from build123d import *

# Parameters (mm, degrees)
SKETCH_1_W               = 5
SKETCH_1_H               = 115
EXTRUDE_1_DEPTH          = 30
EXTRUDE_1_2_DEPTH        = 30
SKETCH_1_3_W             = 37.4
SKETCH_1_3_H             = 115
SKETCH_1_3_W_2           = 30.2
SKETCH_1_3_W_3           = 5
EXTRUDE_2_DEPTH          = 5
CUT_EXTRUDE_1_DEPTH      = 22.5
RIB_1_REACH              = 88.675
SKETCH_4_WALL_W          = 214.94733798
SKETCH_4_WALL_H          = 5
RIB_2_REACH              = 119.1
SKETCH_7_WALL_W          = 265.932906068
SKETCH_7_WALL_H          = 5
MIRROR_3_COPY_1_REACH    = 119.1
MIRROR_3_COPY_1_SKETCH_W = 265.932906068
MIRROR_3_COPY_1_SKETCH_H = 5


with BuildPart() as part:
    # Sketch 1 → Extrude 1 (new body)
    with BuildSketch(Plane.XY):
        with Locations((-17.6, 0)):
            Rectangle(SKETCH_1_W, SKETCH_1_H)
    extrude(amount=-EXTRUDE_1_DEPTH)



with BuildPart() as body_2:
    # Sketch 1 → Extrude 1 2 (new body)
    with BuildSketch(Plane.XY):
        with Locations((17.6, 0)):
            Rectangle(SKETCH_1_W, SKETCH_1_H)
    extrude(amount=-EXTRUDE_1_2_DEPTH)


with BuildPart() as part_1:
    add(part.part)

    add(body_2.part)  # Extrude 2 merges body 2
    # Sketch 1_3 → Extrude 2 (add)
    with BuildSketch(Plane.XY):
        with Locations((-38.8, 0)):
            Rectangle(SKETCH_1_3_W, SKETCH_1_3_H)
        Rectangle(SKETCH_1_3_W_2, SKETCH_1_3_H)
        with Locations((-17.6, 0)):
            Rectangle(SKETCH_1_3_W_3, SKETCH_1_3_H)
        with Locations((17.6, 0)):
            Rectangle(SKETCH_1_3_W_3, SKETCH_1_3_H)
        with Locations((38.8, 0)):
            Rectangle(SKETCH_1_3_W, SKETCH_1_3_H)
    extrude(amount=EXTRUDE_2_DEPTH)

    # Sketch 3 → Cut-Extrude 1 (cut, symmetric)
    with BuildSketch(Plane(origin=(0, 0, 0), x_dir=(0, 0, -1), z_dir=(1, 0, 0))):
        with BuildLine():
            Line((15, 24), (30, 24))
            Line((30, 24), (30, 16))
            Line((30, 16), (15, 16))
            ThreePointArc((15, 16), (11, 20), (15, 24))
        make_face()
        with BuildLine():
            Line((30, -16), (30, -24))
            Line((30, -24), (15, -24))
            ThreePointArc((15, -24), (11, -20), (15, -16))
            Line((15, -16), (30, -16))
        make_face()
    extrude(amount=CUT_EXTRUDE_1_DEPTH, both=True, mode=Mode.SUBTRACT)

    # Sketch 4 wall → Rib 1 (add, up to next)
    with BuildSketch(Plane(origin=(34, 0, -14), x_dir=(0.707106781187, 0, 0.707106781187), z_dir=(0.707106781187, 0, -0.707106781187)), mode=Mode.PRIVATE) as rib_1_sk1:
        Rectangle(SKETCH_4_WALL_W, SKETCH_4_WALL_H)
    rib_1_tool1 = extrude(rib_1_sk1.sketch, amount=-RIB_1_REACH, mode=Mode.PRIVATE) - part_1.part
    rib_1 = rib_1_tool1.solids().sort_by_distance((34, 0, -14))[0]
    add(rib_1)

    # Sketch 7 wall → Rib 2 (add, up to next)
    with BuildSketch(Plane(origin=(25, 40, -14), x_dir=(0.336336396998, 0, 0.941741911595), z_dir=(0.941741911595, 0, -0.336336396998)), mode=Mode.PRIVATE) as rib_2_sk1:
        Rectangle(SKETCH_7_WALL_W, SKETCH_7_WALL_H)
    rib_2_tool1 = extrude(rib_2_sk1.sketch, amount=-RIB_2_REACH, mode=Mode.PRIVATE) - part_1.part
    rib_2 = rib_2_tool1.solids().sort_by_distance((25, 40, -14))[0]
    add(rib_2)

    # Mirror 1: Rib 1 across plane
    add(rib_1.mirror(Plane.ZY))

    # Mirror 2: Rib 2 across plane
    add(rib_2.mirror(Plane.ZY))

    # Mirror 3: Rib 2 across plane
    add(rib_2.mirror(Plane(origin=(0, 0, 0), x_dir=(0, 0, 1), z_dir=(0, -1, 0))))

    # Mirror 3 copy 1 sketch → Mirror 3 copy 1 (add, up to next)
    with BuildSketch(Plane(origin=(-25, -40, -14), x_dir=(-0.336336396998, 0, 0.941741911595), z_dir=(-0.941741911595, 0, -0.336336396998)), mode=Mode.PRIVATE) as mirror_3_copy_1_sk1:
        Rectangle(MIRROR_3_COPY_1_SKETCH_W, MIRROR_3_COPY_1_SKETCH_H)
    mirror_3_copy_1_tool1 = extrude(mirror_3_copy_1_sk1.sketch, amount=-MIRROR_3_COPY_1_REACH, mode=Mode.PRIVATE) - part_1.part
    add(mirror_3_copy_1_tool1.solids().sort_by_distance((-25, -40, -14))[0])


solid = part_1.part
Model file for the job. Use its own axes, mm. A direction names the side the tool comes from. Coordinates: 2 decimals unless noted, no trailing zeros. Write each loop counter-clockwise with the first axis right and the second up, starting at its lowest first coordinate (ties: lowest second). Pieces come first, ordered by that corner, then holes. Notation, with made-up numbers: (24, 53.5) - (66, 53.5) arc R16 ccw to (66, 74.5) - close; hole circle Ø3 at (-29, 85). An arc over 180 degrees is marked (long way). Write each question's results on one line, items separated by ' | '. Start each with the question number.
1) Cut at B-B (y = 12). Write the cut outline in (x, z), then the cut area to 3 significant figures.
2) 3-axis set-ups, long thin cutter, end or side, ignore diameter. For faces 1 (the face through (24, 37.5, -10)), 2 (the face through (-25, 40, -14)), 3 (the face through (-29, -2.5, -9)), 4 (the face through (-18, 16, -23)): which of +Z, -Z, +X, -X, +Y, -Y reach the whole face in a straight line?
3) Cut at A-A (x = -34). Write the cut outline in (y, z), then the cut area to 3 significant figures.
4) Flat gauge pins, fed straight in: P1, Ø10, axis at x = 30, y = -24, coming from the -Z side; P2, Ø12, axis at x = -31.5, z = -26, coming from the -Y side; P3, Ø8, axis at x = 25.5, z = -10, coming from the -Y side; P4, Ø8.5, axis at x = 32, z = -19, coming from the +Y side. Where does each tip first touch, or does it go through?
5) Probe line 1 along Y through (x, z) = (-21.5, -1); line 2 along X through (y, z) = (-46.5, -3); line 3 along Y through (x, z) = (-24, -22). List the from-to ranges inside material, lowest first. Write a range as from..to.
6) Mould opens along X. For faces 5 (the face through (0, 1, 0)), 6 (the face through (-18, -41, -30)), 7 (the face through (34, 0, -14)) say: pulls with the +X half, pulls with the -X half, needs draft (parallel to the pull), parting line crosses it, or undercut.
7) Cut at D-D (z = -23.5). Count the separate pieces of the cut face and the enclosed holes in it, then the cut area to 3 significant figures.
Returned:
1) outline: (-57.5, 0) - (-20.1, 0) - (-20.1, -30) - (-15.1, -30) - (-15.1, 0) - (15.1, 0) - (15.1, -30) - (20.1, -30) - (20.1, 0) - (57.5, 0) - (57.5, 5) - (-57.5, 5) - close | area: 875 mm^2
2) face 1: -Z, +X | face 2: -Z, -X, +Y | face 3: -Z, -X | face 4: -Z, +X, -X
3) outline: (-57.5, 0) - (-2.5, 0) - (-2.5, -14) - (2.5, -14) - (2.5, 0) - (57.5, 0) - (57.5, 5) - (-57.5, 5) - close | area: 645 mm^2
4) P1: z = 0 | P2: through | P3: y = -42.5 | P4: y = 2.5
5) line 1: -42.5..-37.5, -2.5..2.5, 37.5..42.5 | line 2: -20.1..-15.1, 15.1..20.1 | line 3: -2.5..2.5
6) face 5: undercut | face 6: needs draft | face 7: pulls with the +X half
7) separate pieces: 6 | enclosed holes: 0 | area: 1,060 mm^2
